Source: CAD feature listing. Evaluate the final solid. Frame: model axes, mm. Coordinates: 2 decimals unless noted, no trailing zeros. Loops run counter-clockwise (first coordinate to the right, second up) from the corner with the lowest first, then second, coordinate; pieces in that order, holes last. Notation, with made-up numbers: (7, 15.5) -> (19, 15.5) arc R25 cw to (19, 34.5) -> close; hole circle Ø9 at (-3, 85.5). An arc over 180 degrees is marked (long way). Answer as CSV lines item,"result".
from build123d import *

# Parameters (mm, degrees)
F0_W     = 558.8
F0_H     = 406.4
F1_DEPTH = 50.8
F3_DEPTH = 25.4
F4_SIZE  = 12.7


with BuildPart() as f1:
    # F0 (on Top) → F1 (new body)
    with BuildSketch(Plane.XY):
        Rectangle(F0_W, F0_H)
        Polygon((-171.905909, -139.7), (-193.902955, -177.8), (-237.897045, -177.8), (-259.894091, -139.7), (-237.897045, -101.6), (-193.902955, -101.6), align=None, mode=Mode.SUBTRACT)
        Polygon((259.894091, -139.7), (237.897045, -177.8), (193.902955, -177.8), (171.905909, -139.7), (193.902955, -101.6), (237.897045, -101.6), align=None, mode=Mode.SUBTRACT)
        Polygon((-171.905909, 139.7), (-193.902955, 101.6), (-237.897045, 101.6), (-259.894091, 139.7), (-237.897045, 177.8), (-193.902955, 177.8), align=None, mode=Mode.SUBTRACT)
        Polygon((259.894091, 139.7), (237.897045, 101.6), (193.902955, 101.6), (171.905909, 139.7), (193.902955, 177.8), (237.897045, 177.8), align=None, mode=Mode.SUBTRACT)
    extrude(amount=F1_DEPTH)

    # F2 (on face) → F3 (join)
    with BuildSketch(Plane.XY.offset(50.8)):
        Polygon((-237.897045, 101.6), (-193.902955, 101.6), (-171.905909, 139.7), (-193.902955, 177.8), (-237.897045, 177.8), (-259.894091, 139.7), align=None)
        Polygon((193.902955, 101.6), (237.897045, 101.6), (259.894091, 139.7), (237.897045, 177.8), (193.902955, 177.8), (171.905909, 139.7), align=None)
        Polygon((-237.897045, -177.8), (-193.902955, -177.8), (-171.905909, -139.7), (-193.902955, -101.6), (-237.897045, -101.6), (-259.894091, -139.7), align=None)
        Polygon((193.902955, -177.8), (237.897045, -177.8), (259.894091, -139.7), (237.897045, -101.6), (193.902955, -101.6), (171.905909, -139.7), align=None)
    extrude(amount=-F3_DEPTH)

    # F4
    f4_edges = [f1.edges().sort_by_distance(p)[0] for p in [
        (279.4, 0, 50.8),
        (0, -203.2, 50.8),
        (0, 203.2, 50.8),
        (-279.4, 0, 50.8),
    ]]
    chamfer(f4_edges, length=F4_SIZE)


solid = f1.part
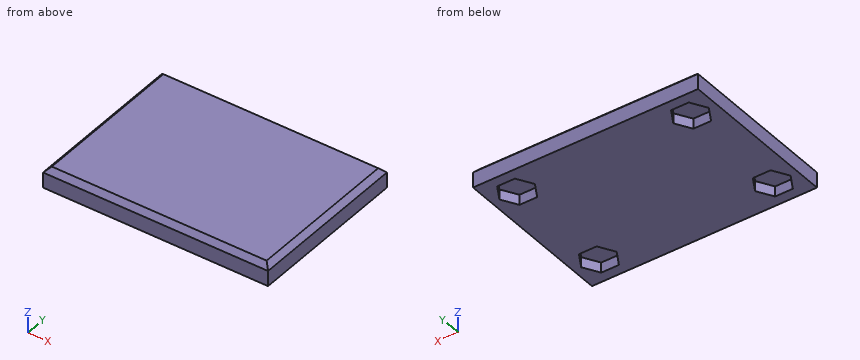
(1) Material intervals for L1, parallel to Y at x = -217.5, z = 23; L2, parallel to X at y = -139.5, z = 23.5; L3, parallel to X at y = -147.5, z = 9.5, sorted ascending. Write a range as [from, to].
Computed values:
L1,"[-203.2, -177.8], [-101.6, 101.6], [177.8, 203.2]"
L2,"[-279.4, -259.78], [-172.02, 172.02], [259.78, 279.4]"
L3,"[-279.4, -255.39], [-176.41, 176.41], [255.39, 279.4]"
(2) Pin query (flat end, axial travel): pin 1 Ø4 at (y, z) = (114.5, 43) entering from +X; pin 2 Ø5 at (x, z) = (187, 44) entering from +Y; pin 3 Ø23 at (x, y) = (-200, 149) entering from -Z. Return the tip coordinate at first contact, or that it passes through.
Computed values:
pin 1,"x = 276.5"
pin 2,"y = 199.8"
pin 3,"z = 25.4"
(3) Cut plane A-A (z = 6). Return the cut outline in (x, y).
Computed values:
outline,"(-279.4, -203.2) -> (279.4, -203.2) -> (279.4, 203.2) -> (-279.4, 203.2) -> close; hole (-259.89, -139.7) -> (-237.9, -177.8) -> (-193.9, -177.8) -> (-171.91, -139.7) -> (-193.9, -101.6) -> (-237.9, -101.6) -> close; hole (-259.89, 139.7) -> (-237.9, 101.6) -> (-193.9, 101.6) -> (-171.91, 139.7) -> (-193.9, 177.8) -> (-237.9, 177.8) -> close; hole (171.91, -139.7) -> (193.9, -177.8) -> (237.9, -177.8) -> (259.89, -139.7) -> (237.9, -101.6) -> (193.9, -101.6) -> close; hole (171.91, 139.7) -> (193.9, 101.6) -> (237.9, 101.6) -> (259.89, 139.7) -> (237.9, 177.8) -> (193.9, 177.8) -> close"
(4) Cut plane C-C (y = 113). Return the cut outline in (x, z).
Computed values:
outline,"(-279.4, 0) -> (-244.48, 0) -> (-244.48, 25.4) -> (-187.32, 25.4) -> (-187.32, 0) -> (187.32, 0) -> (187.32, 25.4) -> (244.48, 25.4) -> (244.48, 0) -> (279.4, 0) -> (279.4, 38.1) -> (266.7, 50.8) -> (-266.7, 50.8) -> (-279.4, 38.1) -> close"
(5) Cut plane B-B (x = 207). Return the cut outline in (y, z), then the cut area to 3 significant figures.
Computed values:
outline,"(-203.2, 0) -> (-177.8, 0) -> (-177.8, 25.4) -> (-101.6, 25.4) -> (-101.6, 0) -> (101.6, 0) -> (101.6, 25.4) -> (177.8, 25.4) -> (177.8, 0) -> (203.2, 0) -> (203.2, 38.1) -> (190.5, 50.8) -> (-190.5, 50.8) -> (-203.2, 38.1) -> close"
area,"16,600 mm^2"
(6) Cut plane D-D (z = 45). Return the cut outline in (x, y), then the cut area to 3 significant figures.
Computed values:
outline,"(-272.5, -196.3) -> (272.5, -196.3) -> (272.5, 196.3) -> (-272.5, 196.3) -> close"
area,"214,000 mm^2"
